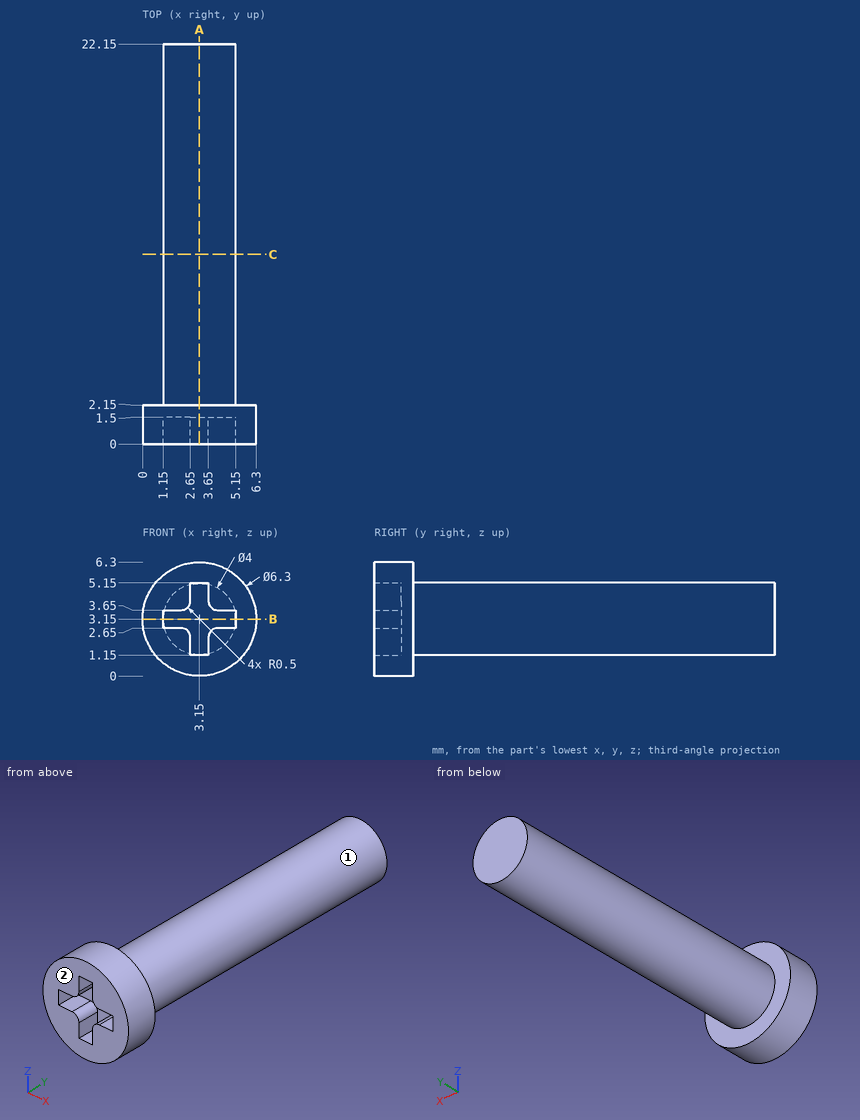
Here's the drawing with two shaded views (mm, measured from the low corner). I have some questions. A direction names the side the tool comes from. Coordinates: 2 decimals unless noted, no trailing zeros. Loops run counter-clockwise (first coordinate to the right, second up) from the corner with the lowest first, then second, coordinate; pieces in that order, holes last. Notation, with made-up numbers: (46, 56) - (68, 56) arc R17 cw to (68, 67) - close; hole circle Ø9 at (47, 74.5). An arc over 180 degrees is marked (long way). Answer as CSV lines item,"result". Start each with the question number.
1) For pin 1 (1.1 mm diameter, centred on x = 2, y = 0.5, fed in from +Z); pin 2 (0.8 mm diameter, centred on y = 1, z = 5, fed in from +X); pin 3 (3 mm diameter, centred on y = 14.5, z = 1.5, fed in from +X), each with a flat end and sliding along its axis, tell me the tip position at first contact or that it passes through.
2) Which directions (+Z, -Z, +X, -X, +Y, -Y) give clear straight access to the entire face, cutting with the end or side of a thin tool? Please do the marked faces 1 and 2.
3) Suppose I cut it at A-A (x = 3.15). Please give me the cut outline in (y, z).
4) I need wall thicknesses on line 1 (Z direction, x = 3.25, y = 11.25); line 2 (Y direction, x = 5.5, z = 2.75); line 3 (Y direction, x = 5, z = 3.5). Which ranges of each line are inside material? Lowest first, please. Write a range as from..to.
5) Suppose I cut it at C-C (y = 10.5). Please give me the cut outline in (x, z).
6) Suppose I cut it at B-B (z = 3.15). Please give me the cut outline in (x, y), plus the area to 3 significant figures.
Check result:
1,pin 1,"stops at z = 6.24"
1,pin 2,"stops at x = 5.95"
1,pin 3,"stops at x = 5.14"
2,face 1,"+Y"
2,face 2,"+Z, -Z, +X, -X, -Y"
3,outline,"(0, 0) - (2.15, 0) - (2.15, 1.15) - (22.15, 1.15) - (22.15, 5.15) - (2.15, 5.15) - (2.15, 6.3) - (0, 6.3) - (0, 5.15) - (1.5, 5.15) - (1.5, 1.15) - (0, 1.15) - close"
4,line 1,"z = 1.15..5.15"
4,line 2,"y = 0..2.15"
4,line 3,"y = 1.5..22.15"
5,outline,"circle Ø4 at (3.15, 3.15)"
6,outline,"(0, 0) - (1.15, 0) - (1.15, 1.5) - (5.15, 1.5) - (5.15, 0) - (6.3, 0) - (6.3, 2.15) - (5.15, 2.15) - (5.15, 22.15) - (1.15, 22.15) - (1.15, 2.15) - (0, 2.15) - close"
6,area,"87.5 mm²"
